CAD build for the part. Positions are in the model's coordinates, mm. Face numbers are marked on the shaded views. Give positions to 0.01 mm unless a question says otherwise; leave off trailing zeros. Order: outer loops, then holes, each group sorted by start corner. A loop starts at its lowest first (then second) coordinate and runs counter-clockwise, first axis right, second up.
from build123d import *


with BuildPart() as f3:
    # F3: sweep along a path in F2
    with BuildLine(Plane.XZ.offset(46.4)) as f3_path:
        ThreePointArc((-101.248391782, 0), (-133.1296067133, 504.0171699309), (-228.2650455746, 1000))
    # F0 (on Top) → F3 (sweep)
    with BuildSketch(Plane.XY):
        with BuildLine():
            Line((161.251608218, 154.3882413845), (-101.248391782, 154.3882413845))
            Line((-101.248391782, 154.3882413845), (-101.248391782, -46.4))
            Line((-101.248391782, -46.4), (-2.2835230583, -46.4))
            Line((-2.2835230583, -46.4), (-2.2835230583, -36.4))
            ThreePointArc((-2.2835230583, -36.4), (18.9296803773, -27.6132034356), (27.7164769417, -6.4))
            Line((27.7164769417, -6.4), (77.7164769417, -6.4))
            Line((77.7164769417, -6.4), (77.7164769417, 35))
            ThreePointArc((77.7164769417, 35), (83.574341318, 49.1421356237), (97.7164769417, 55))
            Line((97.7164769417, 55), (97.7164769417, 65))
            ThreePointArc((97.7164769417, 65), (111.5595193417, 78.7383139253), (116.631133907, 97.5704624512))
            ThreePointArc((116.631133907, 97.5704624512), (130.2645022496, 126.4950867933), (161.251608218, 134.3882413845))
            Line((161.251608218, 134.3882413845), (161.251608218, 154.3882413845))
        make_face()
    sweep(path=f3_path.line)


solid = f3.part
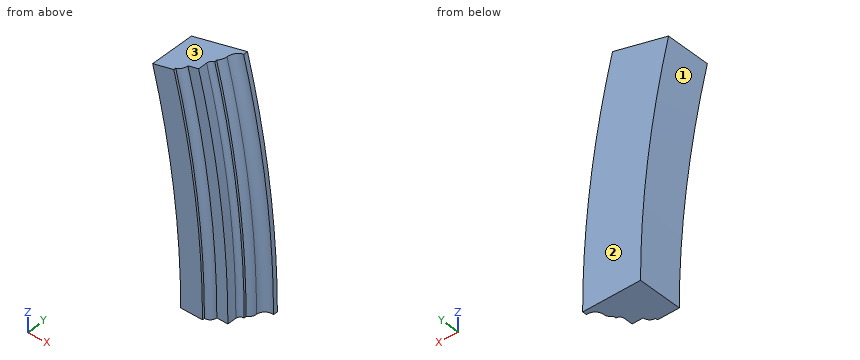
1. Saw through at B-B on x = -189. Give the cut face in (y, z), plus the area to 3 significant figures.
2. Mould opens along Z. For the marked faces 1, 2 and 3 say: released by +Z, released by -Z, zero draft, split by the parting line, or undercut.
3. Saw through at A-A on y = 14.5. Give the cut face in (x, z), plus the area to 3 significant figures.
4. Pin check, flat tips, straight feed: P1, Ø3, axis at y = -25, z = 875, coming from the +X side; P2, Ø3, axis at x = 88.5, z = 390.5, coming from the -Y side. Stop position of each tip, or through.
5. Wall check: line 1 (Y direction, x = -77.5, z = 935.5); line 2 (Y direction, x = 43.5, z = 936); line 3 (Z direction, x = -35, y = 140). Give the ranges that are in metal, low to high.
Reported:
1. outline: (-46.4, 833.25) - (154.39, 833.25) - (154.39, 1010.14) - (-46.4, 1010.14) - close
1. area: 35,500 mm2
2. face 1: released by -Z
2. face 2: zero draft
2. face 3: released by +Z
3. outline: (-228.27, 1000) arc R4000 cw to (-101.25, 0) - (77.72, 0) arc R4178.96 ccw to (-54.98, 1044.74) - close
3. area: 185,000 mm2
4. P1: stops at x = -71.49
4. P2: stops at y = 70.57
5. line 1: y = -6.4 to 154.39
5. line 2: y = 134.54 to 154.39
5. line 3: z = 0 to 1049.9
